Autodesk Inventor part; units mm, degrees
ref_plane "YZ Plane" through (0, 0, 0) normal (1, 0, 0) x (0, 1, 0)
ref_plane "XZ Plane" through (0, 0, 0) normal (0, 1, 0) x (-1, 0, 0)
ref_plane "XY Plane" through (0, 0, 0) normal (0, 0, 1) x (1, 0, 0)
sketch "Sketch1" plane through (0, 0, 0) normal (0, 0, 1) x (1, 0, 0)
  line L0 (-20.85, 0) -> (-20.85, -23)
  line L1 (20.85, -23) -> (20.85, 0)
  line L2 (0, 0) -> (0, -23) construction
  line L3 (-22, 9) -> (-22, 1.15)
  line L4 (-22, 1.15) -> (-20.85, 0)
  line L5 (22, 9) -> (22, 1.15)
  line L6 (22, 1.15) -> (20.85, 0)
  line L7 (0, 0) -> (0, 7.85) construction
  line L8 (-10.6, 9) -> (-9.45, 7.85)
  line L9 (-9.45, 7.85) -> (0, 7.85)
  line L10 (0, 7.85) -> (9.45, 7.85)
  line L11 (9.45, 7.85) -> (10.6, 9)
  line L12 (-22, 9) -> (-10.6, 9)
  line L13 (10.6, 9) -> (22, 9)
  arc A0 (5.5, -18) -> (-5.5, -18) centre (0, -12.1905) ccw
  line L14 (-5.5, -18) -> (5.5, -18) construction
  line L15 (-5.5, -18) -> (-8.8166, -23)
  line L16 (5.5, -18) -> (8.8166, -23)
  line L17 (-20.85, -23) -> (-8.8166, -23)
  line L18 (8.8166, -23) -> (20.85, -23)
  line L19 (8.8166, -23) -> (-8.8166, -23) construction
  arc A1 (8.5116, -22.5401) -> (-8.5116, -22.5401) centre (0, -12.1905) ccw
  point P0 (20.85, -11.5)
  dimension "d1" = 44
  dimension "d3" = 135
  dimension "d4" = 135
  dimension "d5" = 18.9
  dimension "d8" = 23
  dimension "d9" = 135
  dimension "d10" = 23
  dimension "d11" = 1.15
  dimension "d12" = 1.15
  dimension "d13" = 16
  dimension "d14" = 11
  dimension "d16" = 6
  dimension "d17" = 5
  dimension "d18" = 32
  dimension "d19" = 5.4
extrude "Extrusion1" add sketch "Sketch1" along normal mid plane 45.3 contours L4 L3 L12 L8 L9 L10 L11 L13 L5 L6 L1 L18 L16 A1 L15 L17 L0
extrude "Extrusion2" add sketch "Sketch1" along normal mid plane 35.5 contours A1 L16 A0 L15
sketch "Sketch2" plane through (-22, 9, 22.65) normal (0, 1, 0) x (1, 0, 0)
  line L0 (0, 45.3) -> (11.4, 45.3)
  line L1 (0, 45.3) -> (0, 0)
  line L2 (32.6, 45.3) -> (44, 45.3)
  line L3 (44, 45.3) -> (44, 0)
  circle A0 centre (38, 37.65) radius 2.5
  circle A1 centre (38, 7.65) radius 2.5
  line L4 (38, 37.65) -> (38, 7.65) construction
  line L5 (38, 22.65) -> (44, 22.65) construction
  circle A2 centre (6, 37.65) radius 2.5
  circle A3 centre (6, 7.65) radius 2.5
  line L6 (6, 37.65) -> (6, 7.65) construction
  line L7 (6, 22.65) -> (0, 22.65) construction
  point P0 (22, 22.65)
  dimension "d24" = 5
  dimension "d25" = 5
  dimension "d26" = 30
  dimension "d27" = 5
  dimension "d28" = 5
  dimension "d29" = 30
  dimension "d30" = 32
extrude "Extrusion3" cut sketch "Sketch2" against normal blind 15
equation "\"d10\" = d8"
equation "\"d25\" = d24"
equation "\"d28\" = d27"
properties part number "Linear Rail Slider Block"
Input: part model. Units: mm. Frame: model coordinates. A direction names the side the tool comes from. Round coordinates to 2 decimals unless told otherwise and drop trailing zeros. Order: outer loops, then holes, each group sorted by start corner. A loop starts at its lowest first (then second) coordinate and runs counter-clockwise, first axis right, second up. Notation, with made-up numbers: (38, -38.5) - (49, -38.5) arc R19 ccw to (49, -19.5) - close; hole circle Ø8 at (6, 72). An arc over 180 degrees is marked (long way). Answer in a Markdown table with one row per item.
Item 1: Section query C-C (y = 4.5). Return the cut outline in (x, z), then the cut area to 3 significant figures.
Model answer:
| item | result |
|---|---|
| outline | (-22, -22.65) - (22, -22.65) - (22, 22.65) - (-22, 22.65) - close; hole circle Ø5 at (-16, -15); hole circle Ø5 at (-16, 15); hole circle Ø5 at (16, -15); hole circle Ø5 at (16, 15) |
| area | 1,910 mm² |
Item 2: Pin query (flat end, axial travel): pin 1 (6 mm diameter, centred on y = -16.5, z = -10.5, fed in from +X); pin 2 (5.5 mm diameter, centred on x = 17, z = -16, fed in from +Y); pin 3 (1.5 mm diameter, centred on x = -16.5, z = 14, fed in from +Y); pin 4 (10 mm diameter, centred on y = -15, z = 3.5, fed in from -X). Return the tip coordinate at first contact, or that it passes through.
Model answer:
| item | result |
|---|---|
| pin 1 | stops at x = 20.85 |
| pin 2 | stops at y = 9 |
| pin 3 | stops at y = -6 |
| pin 4 | stops at x = -20.85 |
Item 3: Section query B-B (y = -20.5). Return the cut outline in (x, z).
Model answer:
| item | result |
|---|---|
| outline | (-20.85, -22.65) - (-10.51, -22.65) - (-10.51, -17.75) - (-7.16, -17.75) - (-7.16, 17.75) - (-10.51, 17.75) - (-10.51, 22.65) - (-20.85, 22.65) - close; (7.16, -17.75) - (10.51, -17.75) - (10.51, -22.65) - (20.85, -22.65) - (20.85, 22.65) - (10.51, 22.65) - (10.51, 17.75) - (7.16, 17.75) - close |
Item 4: Line query: line 1 (Z direction, x = -16, y = 2.75); line 2 (X direction, y = 2, z = -15); line 3 (X direction, y = -3.5, z = -17). Output: solid intervals per line, ascending.
Model answer:
| item | result |
|---|---|
| line 1 | z = -22.65 to -17.5, -12.5 to 12.5, 17.5 to 22.65 |
| line 2 | x = -22 to -18.5, -13.5 to 13.5, 18.5 to 22 |
| line 3 | x = -20.85 to -17.5, -14.5 to 14.5, 17.5 to 20.85 |
Item 5: Section query A-A (z = -15). Return the cut outline in (x, y), then the cut area to 3 significant figures.
Model answer:
| item | result |
|---|---|
| outline | (-22, 1.15) - (-20.85, 0) - (-20.85, -23) - (-8.82, -23) - (-5.5, -18) arc R8 cw (long way) to (5.5, -18) - (8.82, -23) - (20.85, -23) - (20.85, 0) - (22, 1.15) - (22, 9) - (18.5, 9) - (18.5, -6) - (13.5, -6) - (13.5, 9) - (10.6, 9) - (9.45, 7.85) - (-9.45, 7.85) - (-10.6, 9) - (-13.5, 9) - (-13.5, -6) - (-18.5, -6) - (-18.5, 9) - (-22, 9) - close |
| area | 925 mm² |
Item 6: Section query D-D (x = 0). Return the cut outline in (y, z), then the cut area to 3 significant figures.
Model answer:
| item | result |
|---|---|
| outline | (-4.19, -17.75) - (1.21, -17.75) - (1.21, -22.65) - (7.85, -22.65) - (7.85, 22.65) - (1.21, 22.65) - (1.21, 17.75) - (-4.19, 17.75) - close |
| area | 493 mm² |
Item 7: Mould query, pull axis Z, two halves, no side actions, for faces 6 (the flat face through (16, -6, -15)), 7 (the cylindrical face through (-0.5, 1.2, 20.2)), 8 (the flat face through (0, -3, 17.75)). Classes: released by +Z, released by -Z, zero draft, split by the parting line, or undercut.
Model answer:
| item | result |
|---|---|
| face 6 | undercut |
| face 7 | zero draft |
| face 8 | released by +Z |
Item 8: Reachability of faces 1 (the flat face through (-7.135, -20.465, -0.317)), 2 (the flat face through (10, 8.4, -0.3)), 3 (the flat face through (-16, -6, 15)), 4 (the flat face through (20.85, -12, 0)), 5 (the cylindrical face through (-0.5, 1.2, -20.2)) from +Z, -Z, +X, -X, +Y, -Y: full face, straight path, thin tool, end or side. Return the list, or none.
Model answer:
| item | result |
|---|---|
| face 1 | +Z, -Z, -Y |
| face 2 | +Z, -Z, +Y |
| face 3 | +Y |
| face 4 | +Z, -Z, +X, -Y |
| face 5 | -Z |
